Model file for the job. Use its own axes, mm. Face numbers are marked on the shaded views. A direction names the side the tool comes from. Give positions to 0.01 mm unless a question says otherwise; leave off trailing zeros. Loops run counter-clockwise (first coordinate to the right, second up) from the corner with the lowest first, then second, coordinate; pieces in that order, holes last. Notation, with made-up numbers: M 25,84 L 79,84 A18 cw 79,92 Z; hole C -15.75,27 d1. An arc over 180 degrees is marked long. Answer in a Markdown table with one row per item.
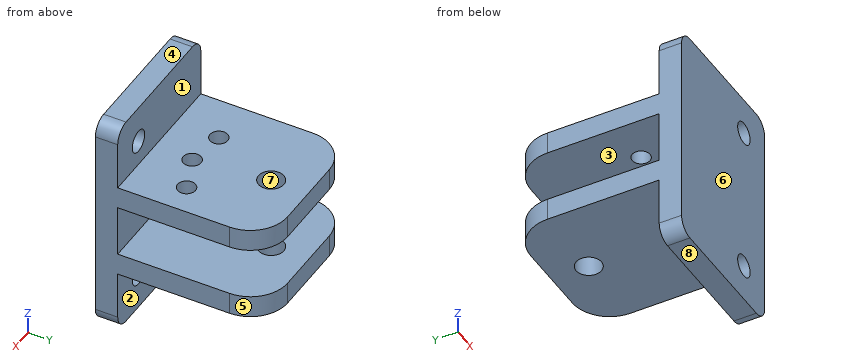
Autodesk Inventor part; units mm, degrees
ref_plane "YZ Plane" through (0, 0, 0) normal (1, 0, 0) x (0, 1, 0)
ref_plane "XZ Plane" through (0, 0, 0) normal (0, 1, 0) x (-1, 0, 0)
ref_plane "XY Plane" through (0, 0, 0) normal (0, 0, 1) x (1, 0, 0)
sketch "Szkic1" plane through (0, 0, 0) normal (0, 1, 0) x (-1, 0, 0)
  line L0 (15, 15) -> (-5, 15)
  line L1 (-5, 15) -> (-5, -15)
  line L2 (-5, -15) -> (15, -15)
  line L3 (15, -15) -> (15, 15)
  point P0 (0, 0)
  point P1 (0, 10)
  point P2 (0, -10)
  dimension "d0" = 20
  dimension "d1" = 20
  dimension "d2" = 15
  dimension "d3" = 5
  dimension "d4" = 5
extrude "Wyciągnięcie proste1" add sketch "Szkic1" along normal blind 3
hole "Otwór1" at (0, 0, 10) at (0, 0, -10) direction (0, 1, 0) diameter 3 end through all
sketch "Szkic2" plane through (0, 3, 0) normal (0, 1, 0) x (1, 0, 0)
  circle A0 centre (0, -10) radius 1.5
  circle A1 centre (0, 10) radius 1.5
  line L0 (-15, -15) -> (5, -15)
  line L1 (5, -15) -> (5, 15)
  line L2 (5, 15) -> (-15, 15)
  line L3 (-15, 15) -> (-15, -15)
  line L4 (5, -15) -> (5, 15)
  line L5 (-15, -6.5) -> (5, -6.5)
  line L6 (5, -6.5) -> (5, -3.5)
  line L7 (5, -3.5) -> (-15, -3.5)
  line L8 (-15, -3.5) -> (-15, -6.5)
  line L9 (-15, 15) -> (-15, -15)
  line L10 (-15, 6.5) -> (5, 6.5)
  line L11 (5, 6.5) -> (5, 3.5)
  line L12 (5, 3.5) -> (-15, 3.5)
  line L13 (-15, 3.5) -> (-15, 6.5)
  point P0 (0, 0)
  dimension "d14" = 3
  dimension "d15" = 3
  dimension "d16" = 2
  dimension "d17" = 2
fillet "Zaokrąglenie1" radius 2 4 edges at (5, 1.5, 15) (-15, 1.5, 15) (5, 1.5, -15) (-15, 1.5, -15)
extrude "Wyciągnięcie proste2" add sketch "Szkic2" along normal blind 20 contours L3 L7 L1 L5 | L3 L10 L1 L12
fillet "Zaokrąglenie2" radius 5 4 edges at (-15, 23, 5) (5, 23, 5) (5, 23, -5) (-15, 23, -5)
sketch "Szkic3" plane through (-15, 3, 6.5) normal (0, 0, 1) x (1, 0, 0)
  arc A0 (5, 20) -> (0, 15) centre (5, 15) ccw
  line L0 (0, 0) -> (0, 15)
  line L1 (20, 0) -> (0, 0)
  line L2 (20, 0) -> (20, 15)
  arc A1 (20, 15) -> (15, 20) centre (15, 15) ccw
  line L3 (5, 20) -> (15, 20)
  point P0 (15, -3)
  point P1 (10, 15)
  dimension "d52" = 10
hole "Otwór2" at (-5, 18, 6.5) direction (0, 0, -1) diameter 3.4 end through all
sketch "Szkic4" plane through (-15, 3, 6.5) normal (0, 0, 1) x (1, 0, 0)
  arc A0 (5, 20) -> (0, 15) centre (5, 15) ccw
  line L0 (0, 0) -> (0, 15)
  line L1 (20, 0) -> (0, 0)
  line L2 (20, 0) -> (20, 15)
  circle A1 centre (10, 15.0001) radius 10 construction
  arc A2 (20, 15) -> (15, 20) centre (15, 15) ccw
  line L3 (5, 20) -> (15, 20)
  point P0 (15, -3)
  point P1 (6.0718, 5.804)
  point P2 (16, 7.0001)
  point P3 (11.1962, 5.0719)
  dimension "d33" = 20
  dimension "d53" = 30
  dimension "d54" = 30
  dimension "d62" = 4
hole "Otwór5" at (-8.9282, 8.804, 6.5) at (1, 10.0001, 6.5) at (-3.8038, 8.0719, 6.5) direction (0, 0, -1) diameter 2.4 end up to surface
sketch "Szkic5" plane through (-15, 3, 6.5) normal (0, 0, 1) x (1, 0, 0)
  circle A0 centre (0, 0) radius 55 construction
  circle A1 centre (137.9996, 0.347) radius 55 construction
  circle A2 centre (275.9991, 0.6941) radius 55 construction
  line L0 (-173.3991, 195.8773) -> (-173.4121, 201.0636) construction
  line L1 (-173.3991, 247) -> (-173.3991, -116) construction
  line L2 (275.9991, -54.3059) -> (-673, -54.3059) construction
  line L3 (-488.3991, -4.3059) -> (-438.3991, -4.3059) construction
  line L4 (-438.3991, -4.3059) -> (-438.3991, -54.3059) construction
  line L5 (-438.3991, -54.3059) -> (-488.3991, -54.3059) construction
  line L6 (-488.3991, -54.3059) -> (-488.3991, -4.3059) construction
  line L7 (-438.4326, 222.6941) -> (233, 222.6941) construction
  line L8 (-438.4326, 192.6941) -> (378, 192.6941) construction
  line L9 (-476, 207.6941) -> (256, 207.6941) construction
  point P0 (15, -3)
  dimension "d63" = 50
  dimension "d64" = 50
  dimension "d65" = 265
  dimension "d66" = 277
  dimension "d67" = 30
  dimension "d68" = 15
equation "\"d15\" = d14"
equation "\"d68\" = 0.5 * d67"
Q1. Saw through at C-C (z = -10). Give the cut face in (x, y).
Reported:
| item | result |
|---|---|
| outline | M -15,0 L -1.5,0 L -1.5,3 L -15,3 Z; M 1.5,0 L 5,0 L 5,3 L 1.5,3 Z |
Q2. Mould opens along Y. For the marked faces 5, 6, 7 and 8 say: released by +Y, released by -Y, zero draft, split by the parting line, or undercut.
Reported:
| item | result |
|---|---|
| face 5 | released by +Y |
| face 6 | released by -Y |
| face 7 | undercut |
| face 8 | zero draft |
Q3. Saw through at B-B (y = 2). Give the cut face in (x, z).
Reported:
| item | result |
|---|---|
| outline | M -15,-13 A2 ccw -13,-15 L 3,-15 A2 ccw 5,-13 L 5,13 A2 ccw 3,15 L -13,15 A2 ccw -15,13 Z; hole C 0,-10 d3; hole C 0,10 d3 |
Q4. Saw through at D-D (x = 1). Give the cut face in (y, z).
Reported:
| item | result |
|---|---|
| outline | M 0,-15 L 3,-15 L 3,-11.12 L 0,-11.12 Z; M 0,-8.88 L 3,-8.88 L 3,-6.5 L 22.9,-6.5 L 22.9,-3.5 L 3,-3.5 L 3,3.5 L 8.8,3.5 L 8.8,6.5 L 3,6.5 L 3,8.88 L 0,8.88 Z; M 0,11.12 L 3,11.12 L 3,15 L 0,15 Z; M 11.2,3.5 L 22.9,3.5 L 22.9,6.5 L 11.2,6.5 Z |
Q5. 3-axis set-ups, long thin cutter, end or side, ignore diameter. For the marked faces 1, 2, 3 and 4: which of +Z, -Z, +X, -X, +Y, -Y reach the whole face in a straight line?
Reported:
| item | result |
|---|---|
| face 1 | +Z, +X, -X, +Y |
| face 2 | -Z, +X, -X, +Y |
| face 3 | +X, -X, +Y |
| face 4 | +Z, +X, -X, +Y, -Y |
Q6. Drop flat-ended pins along their axis: pin 1 (6 mm diameter, centred on x = -1, y = 8.5, fed in from -Z); pin 2 (1 mm diameter, centred on x = 1, y = 16.5, fed in from +Z); pin 3 (1.9 mm diameter, centred on x = 1, y = 10, fed in from +Z). Give the stop position or say it passes through.
Reported:
| item | result |
|---|---|
| pin 1 | z = -6.5 |
| pin 2 | z = 6.5 |
| pin 3 | z = -3.5 |
Q7. Probe probe 1 along Z at (x, y) = (0, 1.95); probe 2 along Y at (x, z) = (-5, -4.75); probe 3 along X at (y, z) = (0.9, -10). List the from-to ranges inside material, lowest first.
Reported:
| item | result |
|---|---|
| probe 1 | -15 to -11.5, -8.5 to 8.5, 11.5 to 15 |
| probe 2 | 0 to 16.3, 19.7 to 23 |
| probe 3 | -15 to -1.5, 1.5 to 5 |
Q8. Saw through at A-A (z = -5.5). Give the cut face in (x, y).
Reported:
| item | result |
|---|---|
| outline | M -15,0 L 5,0 L 5,18 A5 ccw 0,23 L -10,23 A5 ccw -15,18 Z; hole C -5,18 d3.4 |
